Read the model definition and answer for the solid it produces. Units are mm, in the model's axes. Face numbers are marked on the shaded views. Coordinates: 2 decimals unless noted, no trailing zeros. Loops run counter-clockwise (first coordinate to the right, second up) from the corner with the lowest first, then second, coordinate; pieces in that order, holes last. Notation, with made-up numbers: (19, -36) -> (64, -36) arc R13 ccw to (64, -27) -> close; hole circle Ø2 at (84.5, -17). An arc over 180 degrees is marked (long way). Answer as a JSON object with one key per item and string values. Group by question number.
1) Section B-B, the plane x = 0 is taken. Give the vertices of the cut face in (y, z).
2) Section A-A, the plane z = -15.5 is taken. Give the vertices of the cut face in (x, y).
3) Consider probe 1 along Y at (x, z) = (0, -12.5); probe 2 along Y at (x, z) = (-9.5, -8); probe 3 along X at (y, z) = (1, -5.5). Determine where each line is inside the solid, lowest interval first. Write a range as [from, to].
4) Determine the mould class of the marked faces 1, 2, 3 and 4 for opening direction Y: released by +Y, released by -Y, zero draft, split by the parting line, or undercut.
5) A flat-ended cylindrical pin translates along its axis: P1, Ø6, axis at x = 1, y = 9, coming from the -Z side. Find the tip coordinate at first contact, or state that the pin passes through.
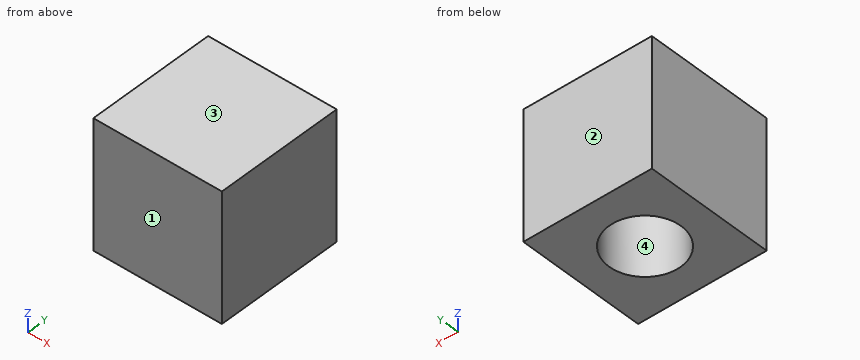
from build123d import *

# Parameters (mm, degrees)
F0_W     = 40
F0_H     = 40
F1_DEPTH = 20
F2_D     = 22.3266
F2_DEPTH = 20.001


with BuildPart() as f1:
    # F0 (on Top) → F1 (new body, symmetric)
    with BuildSketch(Plane.XY):
        Rectangle(F0_W, F0_H)
    extrude(amount=F1_DEPTH, both=True)

    # F2 (through all, one way)
    with BuildSketch(Plane.XY):
        with Locations((0, 0)):
            Circle(F2_D / 2)
    extrude(amount=-F2_DEPTH, mode=Mode.SUBTRACT)


solid = f1.part
Determined:
{
 "1": {"outline": "(-20, -20) -> (-11.16, -20) -> (-11.16, 0) -> (11.16, 0) -> (11.16, -20) -> (20, -20) -> (20, 20) -> (-20, 20) -> close"},
 "2": {"outline": "(-20, -20) -> (20, -20) -> (20, 20) -> (-20, 20) -> close; hole circle Ø22.33 at (0, 0)"},
 "3": {"probe 1": "[-20, -11.16], [11.16, 20]", "probe 2": "[-20, -5.86], [5.86, 20]", "probe 3": "[-20, -11.12], [11.12, 20]"},
 "4": {"face 1": "released by -Y", "face 2": "released by +Y", "face 3": "zero draft", "face 4": "undercut"},
 "5": {"P1": "z = -20"}
}
